Geometry: final body of the model. Coordinates: model frame, mm. A direction names the side the tool comes from. Round coordinates to 2 decimals unless told otherwise and drop trailing zeros. Order: outer loops, then holes, each group sorted by start corner. A loop starts at its lowest first (then second) coordinate and runs counter-clockwise, first axis right, second up. Notation, with made-up numbers: (69, -26) - (83, -26) arc R32 cw to (83, 1) - close; hole circle Ø2 at (-33, 63). An arc over 180 degrees is marked (long way). Put each result on its own line as item: value. Start each with the question number.
(1) Section C-C (x = -47.5). Output: boundary loops of the cut face in (y, z).
(2) Material intervals for L1, parallel to Y at x = 0, z = 10.75 (3 decimals); L2, parallel to Y at x = 51, z = 2; L3, parallel to Y at x = 40, z = 5.25, sorted ascending. Write a range as [from, to].
(3) Access query for faces 1 (the face through (-55.3, 24.594, 8.348)), 2 (the face through (31.24, -54.76, 8.35)). Directions: +Z, -Z, +X, -X, +Y, -Y. A direction counts if a zero-diameter tool reaches every point of the face in a straight line with its end or side. Return the directions, or none.
(4) Section B-B (y = 0). Output: boundary loops of the cut face in (x, z) (3 decimals), and give its area (3 significant figures).
(5) Pull-direction query (X, two-part tool) for faces 3 (the face through (71.49, -26.38, 8.35)), 4 (the face through (-71.424, -26.553, 8.348)), 5 (the face through (32.534, -18.944, 8.348)); classes: released by +X, released by -X, zero draft, split by the parting line, or undercut.
(6) Section D-D (y = -22.5). Output: boundary loops of the cut face in (x, z).
(7) Section A-A (x = 0). Output: boundary loops of the cut face in (y, z) (3 decimals).
(8) Pin query (flat end, axial travel): P1, Ø10, axis at x = 19, z = 2.5, coming from the +Y side; P2, Ø6, axis at x = -16, z = 13.5, coming from the +Y side; P3, Ø5, axis at y = -10.5, z = 1.5, coming from the -X side. Return the tip coordinate at first contact, or that it passes through.
Autodesk Inventor part; units mm, degrees
ref_plane "YZ Plane" through (0, 0, 0) normal (1, 0, 0) x (0, 1, 0)
ref_plane "XZ Plane" through (0, 0, 0) normal (0, 1, 0) x (-1, 0, 0)
ref_plane "XY Plane" through (0, 0, 0) normal (0, 0, 1) x (1, 0, 0)
sketch "Sketch2" plane through (0, 0, 0) normal (0, 0, 1) x (1, 0, 0)
  line L0 (0, 0) -> (87.9881, 0) construction
  line L1 (0, 0) -> (65.9905, 38.1011) construction
  line L2 (65.9905, 38.1011) -> (87.9881, 0) construction
  circle A0 centre (0, 0) radius 76.2 construction
  line L3 (62.5859, 43.4678) -> (34.9256, 27.4975)
  line L4 (68.9361, 32.4694) -> (41.2758, 16.4991)
  arc A1 (34.9256, 27.4975) -> (41.2758, 16.4991) centre (38.1007, 21.9983) ccw
  arc A2 (73.4536, 20.2735) -> (73.4536, -20.2735) centre (87.9881, 0) ccw
  arc A3 (73.4536, 20.2735) -> (68.9361, 32.4694) centre (0, 0) ccw
  line L5 (62.5873, -43.4657) -> (34.9265, -27.4963)
  arc A4 (41.2764, -16.4977) -> (34.9265, -27.4963) centre (38.1014, -21.997) ccw
  line L6 (68.9371, -32.4671) -> (41.2764, -16.4977)
  arc A5 (54.2842, -53.4759) -> (62.5873, -43.4657) centre (0, 0) ccw
  arc A6 (54.2842, -53.4759) -> (19.1694, -73.7494) centre (43.9941, -76.2) ccw
  line L7 (-6.3487, -75.9351) -> (-6.3493, -43.9954)
  arc A7 (6.3507, -43.9952) -> (-6.3493, -43.9954) centre (0.0007, -43.9953) ccw
  line L8 (6.3513, -75.9348) -> (6.3507, -43.9952)
  arc A8 (-19.1694, -73.7494) -> (-6.3487, -75.9351) centre (0, 0) ccw
  arc A9 (-19.1694, -73.7494) -> (-54.2842, -53.4759) centre (-43.9941, -76.2) ccw
  line L9 (-68.9361, -32.4694) -> (-41.2758, -16.4991)
  arc A10 (-34.9256, -27.4975) -> (-41.2758, -16.4991) centre (-38.1007, -21.9983) ccw
  line L10 (-62.5859, -43.4678) -> (-34.9256, -27.4975)
  arc A11 (-73.4536, -20.2735) -> (-68.9361, -32.4694) centre (0, 0) ccw
  arc A12 (-73.4536, -20.2735) -> (-73.4536, 20.2735) centre (-87.9881, 0) ccw
  line L11 (-62.5873, 43.4657) -> (-34.9265, 27.4963)
  arc A13 (-41.2764, 16.4977) -> (-34.9265, 27.4963) centre (-38.1014, 21.997) ccw
  line L12 (-68.9371, 32.4671) -> (-41.2764, 16.4977)
  arc A14 (-54.2842, 53.4759) -> (-62.5873, 43.4657) centre (0, 0) ccw
  arc A15 (-54.2842, 53.4759) -> (-19.1694, 73.7494) centre (-43.9941, 76.2) ccw
  line L13 (6.3487, 75.9351) -> (6.3493, 43.9954)
  arc A16 (-6.3507, 43.9952) -> (6.3493, 43.9954) centre (-0.0007, 43.9953) ccw
  line L14 (-6.3513, 75.9348) -> (-6.3507, 43.9952)
  arc A17 (19.1694, 73.7494) -> (6.3487, 75.9351) centre (0, 0) ccw
  arc A18 (19.1694, 73.7494) -> (54.2842, 53.4759) centre (43.9941, 76.2) ccw
  arc A19 (62.5859, 43.4678) -> (54.2842, 53.4759) centre (0, 0) ccw
  arc A20 (-6.3513, 75.9348) -> (-19.1694, 73.7494) centre (0, 0) ccw
  arc A21 (-68.9371, 32.4671) -> (-73.4536, 20.2735) centre (0, 0) ccw
  arc A22 (-62.5859, -43.4678) -> (-54.2842, -53.4759) centre (0, 0) ccw
  arc A23 (6.3513, -75.9348) -> (19.1694, -73.7494) centre (0, 0) ccw
  arc A24 (68.9371, -32.4671) -> (73.4536, -20.2735) centre (0, 0) ccw
  dimension "d6" = 87.9881
  dimension "d7" = 43.9953
  dimension "d8" = 76.2
  dimension "d9" = 12.7
  dimension "d10" = 32.2047
  dimension "d12" = 24.9453
  dimension "d15" = 360
extrude "Extrusion1" add sketch "Sketch2" along normal blind 16.9333
sketch "Sketch3" plane through (0, 0, 16.9333) normal (0, 0, 1) x (1, 0, 0)
  circle A0 centre (0, 0) radius 9.525
  dimension "d19" = 19.05
extrude "Extrusion2" cut sketch "Sketch3" against normal through all
properties part number "Geneva Driven"
Checks:
1. outline: (-51.5, 0) - (-34.76, 0) - (-34.76, 16.93) - (-51.5, 16.93) - close; (-20.09, 0) - (20.09, 0) - (20.09, 16.93) - (-20.09, 16.93) - close; (34.76, 0) - (51.5, 0) - (51.5, 16.93) - (34.76, 16.93) - close
2. L1: y = [-37.645, -9.525], [9.525, 37.645]
2. L2: y = [-52.26, -36.78], [-22.11, 22.11], [36.78, 52.26]
2. L3: y = [-51.58, -30.43], [-15.94, 15.94], [30.43, 51.58]
3. face 1: +Z, -Z
3. face 2: +Z, -Z, -Y
4. outline: (-63.043, 0) - (-9.525, 0) - (-9.525, 16.933) - (-63.043, 16.933) - close; (9.525, 0) - (63.043, 0) - (63.043, 16.933) - (9.525, 16.933) - close
4. area: 1,810 mm²
5. face 3: released by +X
5. face 4: released by -X
5. face 5: undercut
6. outline: (-72.8, 0) - (-51.67, 0) - (-51.67, 16.93) - (-72.8, 16.93) - close; (-31.77, 0) - (31.77, 0) - (31.77, 16.93) - (-31.77, 16.93) - close; (51.67, 0) - (72.8, 0) - (72.8, 16.93) - (51.67, 16.93) - close
7. outline: (-37.645, 0) - (-9.525, 0) - (-9.525, 16.933) - (-37.645, 16.933) - close; (9.525, 0) - (37.645, 0) - (37.645, 16.933) - (9.525, 16.933) - close
8. P1: stops at y = 74.9
8. P2: stops at y = 75.08
8. P3: stops at x = -66.7
